Read the model definition and answer for the solid it produces. Units are mm, in the model's axes. A direction names the side the tool comes from. Give positions to 0.01 mm unless a question says otherwise; leave off trailing zeros. Write each loop counter-clockwise with the first axis right and the second up, starting at its lowest first coordinate (ties: lowest second). Pieces come first, ordered by that corner, then holes. Notation, with made-up numbers: (-17, 25.25) -> (21, 25.25) arc R8 ccw to (21, 37.25) -> close; hole circle Ø6 at (84, 18.5). An arc over 180 degrees is marked (long way). Answer as CSV lines item,"result". Start each with the question number.
1. A tool of negligible diameter and unlimited length cuts with its end or side. For faces 4 (the flat face through (-7, 12.7, 0)), 5 (the flat face through (-1.25, 12, 0)), 6 (the flat face through (-2, 10.789, 0)), from which of +Z, -Z, +X, -X, +Y, -Y can it reach the whole face along a straight path? Write none if from no direction.
2. For a pull along Y with two mould halves and no side action, classify faces 1 (the flat face through (-12.7, 0, 0)), 2 (the flat face through (7, 12.7, 0)), 3 (the flat face through (2, 10.789, 0)) as pulls with the +Y half, pulls with the -Y half, needs draft (parallel to the pull), parting line crosses it, or undercut.
3. The part is cut by section A-A, the plane x = 0. Determine the outline of the cut face in (y, z) (3 decimals).
4. Find the intervals of material crossed by line 1 (X direction, y = 11, z = -1); line 2 (Y direction, x = 1.5, z = 3.25); line 3 (Y direction, x = 2.75, z = 4), in increasing order.
from build123d import *

# Parameters (mm, degrees)
F1_DEPTH = 6.35
F2_R     = 1.27


with BuildPart() as f1:
    # F0 (on Top) → F1 (new body, symmetric)
    with BuildSketch(Plane.XY):
        with BuildLine():
            Line((-12.7, 12.7), (-12.7, -12.7))
            Line((-12.7, -12.7), (12.7, -12.7))
            Line((12.7, -12.7), (12.7, 12.7))
            Line((12.7, 12.7), (1.250322, 12.7))
            Line((1.250322, 12.7), (1.250322, 10.788764))
            Line((1.250322, 10.788764), (3.81, 10.788764))
            Line((3.81, 10.788764), (3.81, 9.525))
            ThreePointArc((3.81, 9.525), (0, 5.715), (-3.81, 9.525))
            Line((-3.81, 9.525), (-3.81, 10.788764))
            Line((-3.81, 10.788764), (-1.250322, 10.788764))
            Line((-1.250322, 10.788764), (-1.250322, 12.7))
            Line((-1.250322, 12.7), (-12.7, 12.7))
        make_face()
    extrude(amount=F1_DEPTH, both=True)

    # F2
    f2_edges = [f1.edges().sort_by_distance(p)[0] for p in [
        (-3.81, 10.788764, 0),
        (3.81, 10.788764, 0),
    ]]
    fillet(f2_edges, radius=F2_R)


solid = f1.part
Results found:
1,face 4,"+Z, -Z, +X, -X, +Y"
1,face 5,"+Z, -Z, +Y"
1,face 6,"+Z, -Z"
2,face 1,"needs draft"
2,face 2,"pulls with the +Y half"
2,face 3,"undercut"
3,outline,"(-12.7, -6.35) -> (5.715, -6.35) -> (5.715, 6.35) -> (-12.7, 6.35) -> close"
4,line 1,"x = -12.7 to -1.25, 1.25 to 12.7"
4,line 2,"y = -12.7 to 6.02, 10.79 to 12.7"
4,line 3,"y = -12.7 to 6.89, 10.77 to 12.7"
